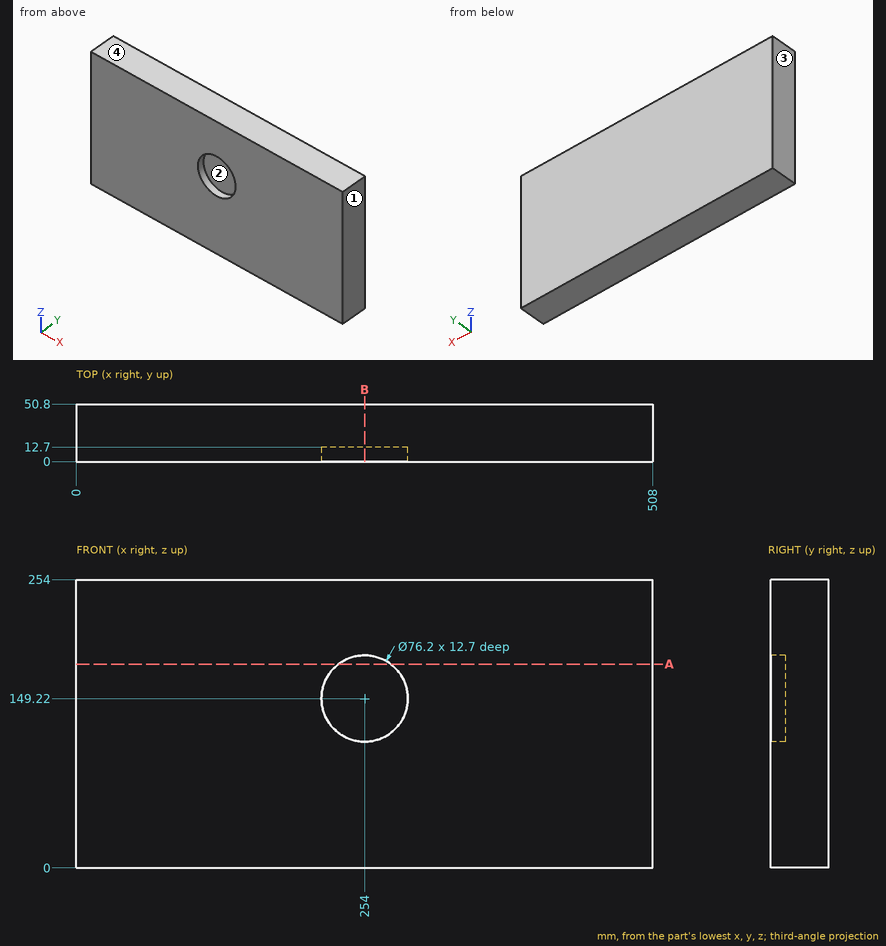
Job drawing, mm, ordinate dimensions from the low corner. One solid piece. Give positions to 0.01 mm unless a question says otherwise; leave off trailing zeros. Loops run counter-clockwise (first coordinate to the right, second up) from the corner with the lowest first, then second, coordinate; pieces in that order, holes last. Notation, with made-up numbers: M -27,-1 L 22,-1 A18 cw 22,13 Z; hole C 34,54.5 d3. An arc over 180 degrees is marked long. Answer in a Markdown table with one row per item. Add a question column.
Item 1: Drop a flat-ended pin along its axis: P1, Ø5, axis at x = 398, y = 42, coming from the -Z side. Give the stop position or say it passes through.
Item 2: Probe probe 1 along Z at (x, y) = (254, 5.25); probe 2 along Z at (x, y) = (260.5, 7). List the from-to ranges inside material, lowest first.
Item 3: Band-saw the part on A-A on z = 179.5. Give the cut face in (x, y).
Item 4: Band-saw the part on B-B on x = 254. Give the cut face in (y, z).
Item 5: Mould opens along X. For the marked faces 1, 2, 3 and 4 say: +X half, -X half, draft (parallel to the pull), parting line (faces both ways), or undercut.
Reply:
| question | item | result |
|---|---|---|
| 1 | P1 | stops at z = 0 |
| 2 | probe 1 | z = 0 to 111.12, 187.32 to 254 |
| 2 | probe 2 | z = 0 to 111.68, 186.76 to 254 |
| 3 | outline | M 0,0 L 230.88,0 L 230.88,12.7 L 277.12,12.7 L 277.12,0 L 508,0 L 508,50.8 L 0,50.8 Z |
| 4 | outline | M 0,0 L 50.8,0 L 50.8,254 L 0,254 L 0,187.32 L 12.7,187.32 L 12.7,111.12 L 0,111.12 Z |
| 5 | face 1 | +X half |
| 5 | face 2 | undercut |
| 5 | face 3 | -X half |
| 5 | face 4 | draft |
